```python
from build123d import *

# Parameters (mm, degrees)
F0_R     = 1.2
F1_DEPTH = 1.5
F2_DEPTH = 5
F3_DEPTH = 5.5
F5_DEPTH = 2
F7_DEPTH = 2


# Not quite as in the source:
# - a feature names something its author has since deleted; it is built from what else it names


with BuildPart() as f1:
    # F0 (on Top) → F1 (new body)
    with BuildSketch(Plane.XY):
        with BuildLine():
            Line((14.9310000289, -10.5), (14.9310000289, 10.5))
            ThreePointArc((14.9310000289, 10.5), (13.4665339264, 14.0355339264), (9.931, 15.5000000289))
            Line((9.931, 15.5000000289), (-9.931, 15.5000000289))
            ThreePointArc((-9.931, 15.5000000289), (-13.4665339264, 14.0355339264), (-14.9310000289, 10.5))
            Line((-14.9310000289, 10.5), (-14.9310000289, -10.5))
            ThreePointArc((-14.9310000289, -10.5), (-13.4665339264, -14.0355339264), (-9.931, -15.5000000289))
            Line((-9.931, -15.5000000289), (9.931, -15.5000000289))
            ThreePointArc((9.931, -15.5000000289), (13.4665339264, -14.0355339264), (14.9310000289, -10.5))
        make_face()
        with BuildLine():
            Line((-9.931, 13.5000000289), (-7.581, 13.5000000289))
            Line((-7.581, 13.5000000289), (0.069, 13.5000000289))
            Line((0.069, 13.5000000289), (4.769, 13.5000000289))
            Line((4.769, 13.5000000289), (9.931, 13.5000000289))
            ThreePointArc((9.931, 13.5000000289), (12.052320364, 12.621320364), (12.9310000289, 10.5))
            Line((12.9310000289, 10.5), (12.9310000289, -10.5))
            ThreePointArc((12.9310000289, -10.5), (12.052320364, -12.621320364), (9.931, -13.5000000289))
            Line((9.931, -13.5000000289), (4.769, -13.5000000289))
            Line((4.769, -13.5000000289), (0.069, -13.5000000289))
            Line((0.069, -13.5000000289), (-7.581, -13.5000000289))
            Line((-7.581, -13.5000000289), (-9.931, -13.5000000289))
            ThreePointArc((-9.931, -13.5000000289), (-12.052320364, -12.621320364), (-12.9310000289, -10.5))
            Line((-12.9310000289, -10.5), (-12.9310000289, -8.1))
            Line((-12.9310000289, -8.1), (-12.9310000289, 8.1))
            Line((-12.9310000289, 8.1), (-12.9310000289, 10.5))
            ThreePointArc((-12.9310000289, 10.5), (-12.052320364, 12.621320364), (-9.931, 13.5000000289))
        make_face(mode=Mode.SUBTRACT)
        with BuildLine():
            ThreePointArc((4.769, -10.45), (2.419, -8.1), (0.069, -10.45))
            ThreePointArc((0.069, -10.45), (2.419, -12.8), (4.769, -10.45))
        make_face()
        with Locations((2.419, -10.45)):
            Circle(F0_R, mode=Mode.SUBTRACT)
        with BuildLine():
            ThreePointArc((4.769, 10.45), (2.419, 12.8), (0.069, 10.45))
            ThreePointArc((0.069, 10.45), (2.419, 8.1), (4.769, 10.45))
        make_face()
        with Locations((2.419, 10.45)):
            Circle(F0_R, mode=Mode.SUBTRACT)
        with BuildLine():
            ThreePointArc((-9.931, 8.1), (-11.5927009358, 12.1117009358), (-7.581, 10.45))
            Line((-7.581, 10.45), (-7.581, 13.5000000289))
            Line((-7.581, 13.5000000289), (-9.931, 13.5000000289))
            ThreePointArc((-9.931, 13.5000000289), (-12.052320364, 12.621320364), (-12.9310000289, 10.5))
            Line((-12.9310000289, 10.5), (-12.9310000289, 8.1))
            Line((-12.9310000289, 8.1), (-9.931, 8.1))
        make_face()
        with BuildLine():
            Line((-9.931, -8.1), (-12.9310000289, -8.1))
            Line((-12.9310000289, -8.1), (-12.9310000289, -10.5))
            ThreePointArc((-12.9310000289, -10.5), (-12.052320364, -12.621320364), (-9.931, -13.5000000289))
            Line((-9.931, -13.5000000289), (-7.581, -13.5000000289))
            Line((-7.581, -13.5000000289), (-7.581, -10.45))
            ThreePointArc((-7.581, -10.45), (-11.5927009358, -12.1117009358), (-9.931, -8.1))
        make_face()
        with BuildLine():
            ThreePointArc((-7.581, -10.45), (-8.2692990642, -8.7882990642), (-9.931, -8.1))
            ThreePointArc((-9.931, -8.1), (-11.5927009358, -12.1117009358), (-7.581, -10.45))
        make_face()
        with Locations((-9.931, -10.45)):
            Circle(F0_R, mode=Mode.SUBTRACT)
        with BuildLine():
            Line((0.069, -10.45), (0.069, -13.5000000289))
            Line((0.069, -13.5000000289), (4.769, -13.5000000289))
            Line((4.769, -13.5000000289), (4.769, -10.45))
            ThreePointArc((4.769, -10.45), (2.419, -12.8), (0.069, -10.45))
        make_face()
        with BuildLine():
            ThreePointArc((-9.931, 8.1), (-8.2692990642, 8.7882990642), (-7.581, 10.45))
            ThreePointArc((-7.581, 10.45), (-11.5927009358, 12.1117009358), (-9.931, 8.1))
        make_face()
        with Locations((-9.931, 10.45)):
            Circle(F0_R, mode=Mode.SUBTRACT)
        with BuildLine():
            Line((4.769, 13.5000000289), (0.069, 13.5000000289))
            Line((0.069, 13.5000000289), (0.069, 10.45))
            ThreePointArc((0.069, 10.45), (2.419, 12.8), (4.769, 10.45))
            Line((4.769, 10.45), (4.769, 13.5000000289))
        make_face()
        with BuildLine():
            Line((-7.581, 13.5000000289), (-7.581, 10.45))
            ThreePointArc((-7.581, 10.45), (-8.2692990642, 8.7882990642), (-9.931, 8.1))
            Line((-9.931, 8.1), (-12.9310000289, 8.1))
            Line((-12.9310000289, 8.1), (-12.9310000289, -8.1))
            Line((-12.9310000289, -8.1), (-9.931, -8.1))
            ThreePointArc((-9.931, -8.1), (-8.2692990642, -8.7882990642), (-7.581, -10.45))
            Line((-7.581, -10.45), (-7.581, -13.5000000289))
            Line((-7.581, -13.5000000289), (0.069, -13.5000000289))
            Line((0.069, -13.5000000289), (0.069, -10.45))
            ThreePointArc((0.069, -10.45), (2.419, -8.1), (4.769, -10.45))
            Line((4.769, -10.45), (4.769, -13.5000000289))
            Line((4.769, -13.5000000289), (9.931, -13.5000000289))
            ThreePointArc((9.931, -13.5000000289), (12.052320364, -12.621320364), (12.9310000289, -10.5))
            Line((12.9310000289, -10.5), (12.9310000289, 10.5))
            ThreePointArc((12.9310000289, 10.5), (12.052320364, 12.621320364), (9.931, 13.5000000289))
            Line((9.931, 13.5000000289), (4.769, 13.5000000289))
            Line((4.769, 13.5000000289), (4.769, 10.45))
            ThreePointArc((4.769, 10.45), (2.419, 8.1), (0.069, 10.45))
            Line((0.069, 10.45), (0.069, 13.5000000289))
            Line((0.069, 13.5000000289), (-7.581, 13.5000000289))
        make_face()
    extrude(amount=F1_DEPTH)

    # F0 (on Top) → F2 (join)
    with BuildSketch(Plane.XY):
        with BuildLine():
            ThreePointArc((-9.931, 8.1), (-11.5927009358, 12.1117009358), (-7.581, 10.45))
            Line((-7.581, 10.45), (-7.581, 13.5000000289))
            Line((-7.581, 13.5000000289), (-9.931, 13.5000000289))
            ThreePointArc((-9.931, 13.5000000289), (-12.052320364, 12.621320364), (-12.9310000289, 10.5))
            Line((-12.9310000289, 10.5), (-12.9310000289, 8.1))
            Line((-12.9310000289, 8.1), (-9.931, 8.1))
        make_face()
        with BuildLine():
            ThreePointArc((-9.931, 8.1), (-8.2692990642, 8.7882990642), (-7.581, 10.45))
            ThreePointArc((-7.581, 10.45), (-11.5927009358, 12.1117009358), (-9.931, 8.1))
        make_face()
        with Locations((-9.931, 10.45)):
            Circle(F0_R, mode=Mode.SUBTRACT)
        with BuildLine():
            ThreePointArc((4.769, 10.45), (2.419, 12.8), (0.069, 10.45))
            ThreePointArc((0.069, 10.45), (2.419, 8.1), (4.769, 10.45))
        make_face()
        with Locations((2.419, 10.45)):
            Circle(F0_R, mode=Mode.SUBTRACT)
        with BuildLine():
            Line((4.769, 13.5000000289), (0.069, 13.5000000289))
            Line((0.069, 13.5000000289), (0.069, 10.45))
            ThreePointArc((0.069, 10.45), (2.419, 12.8), (4.769, 10.45))
            Line((4.769, 10.45), (4.769, 13.5000000289))
        make_face()
        with BuildLine():
            ThreePointArc((4.769, -10.45), (2.419, -8.1), (0.069, -10.45))
            ThreePointArc((0.069, -10.45), (2.419, -12.8), (4.769, -10.45))
        make_face()
        with Locations((2.419, -10.45)):
            Circle(F0_R, mode=Mode.SUBTRACT)
        with BuildLine():
            Line((0.069, -10.45), (0.069, -13.5000000289))
            Line((0.069, -13.5000000289), (4.769, -13.5000000289))
            Line((4.769, -13.5000000289), (4.769, -10.45))
            ThreePointArc((4.769, -10.45), (2.419, -12.8), (0.069, -10.45))
        make_face()
        with BuildLine():
            ThreePointArc((-7.581, -10.45), (-8.2692990642, -8.7882990642), (-9.931, -8.1))
            ThreePointArc((-9.931, -8.1), (-11.5927009358, -12.1117009358), (-7.581, -10.45))
        make_face()
        with Locations((-9.931, -10.45)):
            Circle(F0_R, mode=Mode.SUBTRACT)
        with BuildLine():
            Line((-9.931, -8.1), (-12.9310000289, -8.1))
            Line((-12.9310000289, -8.1), (-12.9310000289, -10.5))
            ThreePointArc((-12.9310000289, -10.5), (-12.052320364, -12.621320364), (-9.931, -13.5000000289))
            Line((-9.931, -13.5000000289), (-7.581, -13.5000000289))
            Line((-7.581, -13.5000000289), (-7.581, -10.45))
            ThreePointArc((-7.581, -10.45), (-11.5927009358, -12.1117009358), (-9.931, -8.1))
        make_face()
    extrude(amount=F2_DEPTH)

    # F0 (on Top) → F3 (join)
    with BuildSketch(Plane.XY):
        with BuildLine():
            Line((14.9310000289, -10.5), (14.9310000289, 10.5))
            ThreePointArc((14.9310000289, 10.5), (13.4665339264, 14.0355339264), (9.931, 15.5000000289))
            Line((9.931, 15.5000000289), (-9.931, 15.5000000289))
            ThreePointArc((-9.931, 15.5000000289), (-13.4665339264, 14.0355339264), (-14.9310000289, 10.5))
            Line((-14.9310000289, 10.5), (-14.9310000289, -10.5))
            ThreePointArc((-14.9310000289, -10.5), (-13.4665339264, -14.0355339264), (-9.931, -15.5000000289))
            Line((-9.931, -15.5000000289), (9.931, -15.5000000289))
            ThreePointArc((9.931, -15.5000000289), (13.4665339264, -14.0355339264), (14.9310000289, -10.5))
        make_face()
        with BuildLine():
            Line((-9.931, 13.5000000289), (-7.581, 13.5000000289))
            Line((-7.581, 13.5000000289), (0.069, 13.5000000289))
            Line((0.069, 13.5000000289), (4.769, 13.5000000289))
            Line((4.769, 13.5000000289), (9.931, 13.5000000289))
            ThreePointArc((9.931, 13.5000000289), (12.052320364, 12.621320364), (12.9310000289, 10.5))
            Line((12.9310000289, 10.5), (12.9310000289, -10.5))
            ThreePointArc((12.9310000289, -10.5), (12.052320364, -12.621320364), (9.931, -13.5000000289))
            Line((9.931, -13.5000000289), (4.769, -13.5000000289))
            Line((4.769, -13.5000000289), (0.069, -13.5000000289))
            Line((0.069, -13.5000000289), (-7.581, -13.5000000289))
            Line((-7.581, -13.5000000289), (-9.931, -13.5000000289))
            ThreePointArc((-9.931, -13.5000000289), (-12.052320364, -12.621320364), (-12.9310000289, -10.5))
            Line((-12.9310000289, -10.5), (-12.9310000289, -8.1))
            Line((-12.9310000289, -8.1), (-12.9310000289, 8.1))
            Line((-12.9310000289, 8.1), (-12.9310000289, 10.5))
            ThreePointArc((-12.9310000289, 10.5), (-12.052320364, 12.621320364), (-9.931, 13.5000000289))
        make_face(mode=Mode.SUBTRACT)
    extrude(amount=F3_DEPTH)

    # F4 (on face) → F5 (cut)
    with BuildSketch(Plane(origin=(-14.9310000289, 0, 0), x_dir=(0, -1, 0), z_dir=(-1, 0, 0))):
        with BuildLine():
            Line((7, 5.5), (-7, 5.5))
            Line((-7, 5.5), (-7, 4.75))
            ThreePointArc((-7, 4.75), (-6.8535533906, 4.3964466094), (-6.5, 4.25))
            Line((-6.5, 4.25), (6.5, 4.25))
            ThreePointArc((6.5, 4.25), (6.8535533906, 4.3964466094), (7, 4.75))
            Line((7, 4.75), (7, 5.5))
        make_face()
    extrude(amount=-F5_DEPTH, mode=Mode.SUBTRACT)

    # F6 (on face) → F7 (cut)
    with BuildSketch(Plane.YZ.offset(14.9310000289)):
        with BuildLine():
            Line((9, 2), (9, 5.5))
            Line((9, 5.5), (-9, 5.5))
            Line((-9, 5.5), (-9, 2))
            ThreePointArc((-9, 2), (-8.8535533906, 1.6464466094), (-8.5, 1.5))
            Line((-8.5, 1.5), (8.5, 1.5))
            ThreePointArc((8.5, 1.5), (8.8535533906, 1.6464466094), (9, 2))
        make_face()
    extrude(amount=-F7_DEPTH, mode=Mode.SUBTRACT)


solid = f1.part
```
Input: part model. Units: mm. Frame: model coordinates. A direction names the side the tool comes from. Give positions to 0.01 mm unless a question says otherwise; leave off trailing zeros. Write each loop counter-clockwise with the first axis right and the second up, starting at its lowest first coordinate (ties: lowest second). Pieces come first, ordered by that corner, then holes. Notation, with made-up numbers: (59, -37.5) - (113, -37.5) arc R25 cw to (113, 0.5) - close; hole circle Ø2 at (-34.5, 81.25). An arc over 180 degrees is marked (long way). Write item = value, one per line. Start each with the question number.
1) Cut plane A-A (y = -10). Return loops of the section in (x, z).
2) Cut plane D-D (z = 3.85). Give the number of separate pieces and of enclosed holes in the cut face, and give its area (3 significant figures).
3) Pin query (flat end, axial travel): pin 1 (2.5 mm diameter, centred on x = -11.5, z = 3.5, fed in from +Y); pin 2 (2 mm diameter, centred on x = 13.5, z = 4.5, fed in from +Y); pin 3 (5 mm diameter, centred on x = 3.5, y = 10, fed in from +Z). Return the tip coordinate at first contact, or that it passes through.
4) Cut plane B-B (x = -5). Return loops of the section in (y, z), and give its area (3 significant figures).
5) Material intervals for L1, parallel to Y at x = 5.5, z = 3.65; L2, parallel to Z at x = 9.5, y = -8; L3, parallel to Y at x = 11.25, z = 3.9, sorted ascending. Write a range as [from, to].
6) Cut plane C-C (y = 2.5). Return loops of the section in (x, z), and give its area (3 significant figures).
7) Reachability of faces 1 (the face through (2, 12, 5)), 2 (the face through (-9.286, -9.438, 2.465)), 3 (the face through (14, 9, 4)) from +Z, -Z, +X, -X, +Y, -Y: full face, straight path, thin tool, end or side. Return the list, or none.
Answers follow:
q1.outline = (-14.93, 0) - (-11.04, 0) - (-11.04, 5) - (-12.93, 5) - (-12.93, 5.5) - (-14.93, 5.5) - close; (-8.82, 0) - (1.31, 0) - (1.31, 5) - (0.11, 5) - (0.11, 1.5) - (-7.62, 1.5) - (-7.62, 5) - (-8.82, 5) - close; (3.53, 0) - (14.93, 0) - (14.93, 5.5) - (12.93, 5.5) - (12.93, 1.5) - (4.73, 1.5) - (4.73, 5) - (3.53, 5) - close
q2.separate_pieces = 1
q2.enclosed_holes = 4
q2.area = 257 mm^2
q3.pin_1 = 15.49
q3.pin_2 = 14.79
q3.pin_3 = 5
q4.outline = (-15.5, 0) - (15.5, 0) - (15.5, 5.5) - (13.5, 5.5) - (13.5, 1.5) - (-13.5, 1.5) - (-13.5, 5.5) - (-15.5, 5.5) - close
q4.area = 62.5 mm^2
q5.L1 = [-15.5, -13.5], [13.5, 15.5]
q5.L2 = [0, 1.5]
q5.L3 = [-15.32, -13.19], [13.19, 15.32]
q6.outline = (-14.93, 0) - (14.93, 0) - (14.93, 1.5) - (-12.93, 1.5) - (-12.93, 4.25) - (-14.93, 4.25) - close
q6.area = 50.3 mm^2
q7.face_1 = +Z
q7.face_2 = +Z, -Z
q7.face_3 = +Z, +X
